Here's how the part is built. I have some questions about the finished solid (model axes, mm). A direction names the side the tool comes from. Round coordinates to 2 decimals unless told otherwise and drop trailing zeros. Order: outer loops, then holes, each group sorted by start corner. A loop starts at its lowest first (then second) coordinate and runs counter-clockwise, first axis right, second up.
```python
from build123d import *

# Parameters (mm, degrees)
SKETCH1_R           = 12.5
BOSS_EXTRUDE1_DEPTH = 67
SKETCH2_R           = 4.5
BOSS_EXTRUDE3_DEPTH = 3
SKETCH3_R           = 3
BOSS_EXTRUDE4_DEPTH = 15.2


with BuildPart() as part:
    # Sketch1 → Boss-Extrude1 (new body)
    with BuildSketch(Plane.XY):
        Circle(SKETCH1_R)
    extrude(amount=BOSS_EXTRUDE1_DEPTH)

    # Sketch2 → Boss-Extrude3 (add)
    with BuildSketch(Plane.XY.offset(67)):
        Circle(SKETCH2_R)
    extrude(amount=BOSS_EXTRUDE3_DEPTH)

    # Sketch3 → Boss-Extrude4 (add)
    with BuildSketch(Plane.XY.offset(70)):
        with Locations(Location((0, 0, 0), (0, 0, 180))):
            Circle(SKETCH3_R)
    extrude(amount=BOSS_EXTRUDE4_DEPTH)


solid = part.part
```
1) If we section it at D-D (y = -7): Write out the boundary of the cut face in (x, z), plus the area to 3 significant figures.
2) I'm going to push flat-ended pins straight in: pin 1 (2 mm diameter, centred on x = 4, z = 67.5, fed in from +Y); pin 2 (1.5 mm diameter, centred on x = -6.5, y = -3, fed in from +Z); pin 3 (4 mm diameter, centred on x = -6, z = 63.5, fed in from -Y); pin 4 (4 mm diameter, centred on y = 0.5, z = 39, fed in from -X). Where does each tip first touch, or does it pass through?
3) I need wall thicknesses on line 1 (Z direction, x = -6, y = 8.75); line 2 (X direction, y = 2.25, z = 53.5); line 3 (Y direction, x = 7.25, z = 65.5). Which ranges of each line are inside material? Lowest first, please.
4) If we section it at A-A (x = 0): Write out the boundary of the cut face in (y, z).
5) If we section it at C-C (z = 63.5): Write out the boundary of the cut face in (x, y), plus the area to 3 significant figures.
6) For faces 1 (the flat face through (0, 0, 85.2)), 2 (the flat face through (0, -5, 67)), which set-ups out of +Z, -Z, +X, -X, +Y, -Y let a thin tool reach every point of the face, with its end or its side?
Solutions:
1. outline: (-10.36, 0) - (10.36, 0) - (10.36, 67) - (-10.36, 67) - close
1. area: 1,390 mm2
2. pin 1: stops at y = 12.1
2. pin 2: stops at z = 67
2. pin 3: stops at y = -11.84
2. pin 4: stops at x = -12.5
3. line 1: z = 0 to 67
3. line 2: x = -12.3 to 12.3
3. line 3: y = -10.18 to 10.18
4. outline: (-12.5, 0) - (12.5, 0) - (12.5, 67) - (4.5, 67) - (4.5, 70) - (3, 70) - (3, 85.2) - (-3, 85.2) - (-3, 70) - (-4.5, 70) - (-4.5, 67) - (-12.5, 67) - close
5. outline: circle Ø25 at (0, 0)
5. area: 491 mm2
6. face 1: +Z, +X, -X, +Y, -Y
6. face 2: +Z
